```python
from build123d import *

# Parameters (mm, degrees)
SKETCH_1_R          = 9.1
EXTRUDE_1_DEPTH     = 64.7
FILLET_1_R          = 0.5
FILLET_2_R          = 0.5
SKETCH_2_R          = 6.5
CUT_EXTRUDE_1_DEPTH = 0.35
SKETCH_3_R          = 6.5
CUT_EXTRUDE_2_DEPTH = 0.35
SKETCH_4_R          = 4.25
EXTRUDE_2_DEPTH     = 0.8
FILLET_3_R          = 0.5
SKETCH_5_R          = 6.5
SKETCH_5_R_2        = 4.25
EXTRUDE_3_DEPTH     = 0.2


with BuildPart() as part:
    # 草图1 → 凸台-拉伸1 (new body)
    with BuildSketch(Plane.XY):
        with Locations((-28.874360447, 15.271996124)):
            Circle(SKETCH_1_R)
    extrude(amount=EXTRUDE_1_DEPTH)

    # 圆角1
    fillet_1_edges = [part.edges().sort_by_distance(p)[0] for p in [
        (-37.974360447, 15.271996124, 0),
    ]]
    fillet(fillet_1_edges, radius=FILLET_1_R)

    # 圆角2
    fillet_2_edges = [part.edges().sort_by_distance(p)[0] for p in [
        (-37.974360447, 15.271996124, 64.7),
    ]]
    fillet(fillet_2_edges, radius=FILLET_2_R)

    # 草图2 → 切除-拉伸1 (cut)
    with BuildSketch(Plane(origin=(0, 0, 0), x_dir=(-1, 0, 0), z_dir=(0, 0, -1))):
        with Locations((28.874360447, 15.271996124)):
            Circle(SKETCH_2_R)
    extrude(amount=-CUT_EXTRUDE_1_DEPTH, mode=Mode.SUBTRACT)

    # 草图3 → 切除-拉伸2 (cut)
    with BuildSketch(Plane.XY.offset(64.7)):
        with Locations((-28.874360447, 15.271996124)):
            Circle(SKETCH_3_R)
    extrude(amount=-CUT_EXTRUDE_2_DEPTH, mode=Mode.SUBTRACT)

    # 草图4 → 凸台-拉伸2 (add)
    with BuildSketch(Plane.XY.offset(64.35)):
        with Locations((-28.874360447, 15.271996124)):
            Circle(SKETCH_4_R)
    extrude(amount=EXTRUDE_2_DEPTH)

    # 圆角3
    fillet_3_edges = [part.edges().sort_by_distance(p)[0] for p in [
        (-33.124360447, 15.271996124, 65.15),
    ]]
    fillet(fillet_3_edges, radius=FILLET_3_R)

    # 草图5 → 凸台-拉伸3 (add)
    with BuildSketch(Plane.XY.offset(64.35)):
        with Locations((-28.874360447, 15.271996124)):
            Circle(SKETCH_5_R)
        with Locations((-28.874360447, 15.271996124)):
            Circle(SKETCH_5_R_2, mode=Mode.SUBTRACT)
    extrude(amount=EXTRUDE_3_DEPTH)


solid = part.part
```
Here's how the part is built. I have some questions about the finished solid (model axes, mm). A direction names the side the tool comes from. Round coordinates to 2 decimals unless told otherwise and drop trailing zeros. Order: outer loops, then holes, each group sorted by start corner. A loop starts at its lowest first (then second) coordinate and runs counter-clockwise, first axis right, second up. Notation, with made-up numbers: M 6,80.25 L 41,80.25 A29 ccw 41,111.25 Z; hole C -21,11 d7. An arc over 180 degrees is marked long. Answer in a Markdown table with one row per item.
Item 1: Imagine slicing it at A-A, the plane z = 49. Write out the boundary of the cut face in (x, y).
A:
| item | result |
|---|---|
| outline | C -28.87,15.27 d18.2 |
Item 2: Thinking about a two-plate mould opening in Y: for faces 4 (the face through (-37.966, 15.672, 31.904)), 5 (the face through (-29, 15, 0.35)), 6 (the face through (-29, 15, 65.15)), which applies, +Y half, -Y half, draft (parallel to the pull), parting line (faces both ways), or undercut?
A:
| item | result |
|---|---|
| face 4 | parting line |
| face 5 | undercut |
| face 6 | draft |
Item 3: For faces 1 (the face through (-28, 22, 0)), 2 (the face through (-22.38, 15.56, 0.17)), 3 (the face through (-28, 22, 64.7)), which set-ups out of +Z, -Z, +X, -X, +Y, -Y let a thin tool reach every point of the face, with its end or its side?
A:
| item | result |
|---|---|
| face 1 | -Z, +X, -X, +Y, -Y |
| face 2 | -Z |
| face 3 | +Z |
Item 4: If I drill on L1, parallel to Z at x = -26, y = 10; L2, parallel to Z at x = -31, y = 12.75; L3, parallel to Y at x = -22.5, z = 23.5, over which ranges is the centre line in solid material (lowest first)? Write a range as from..to.
A:
| item | result |
|---|---|
| L1 | z = 0.35..64.55 |
| L2 | z = 0.35..65.15 |
| L3 | y = 8.78..21.77 |
Item 5: I'm going to push flat-ended pins straight in: pin 1 (1 mm diameter, centred on y = 16, z = 33.5, fed in from -X); pin 2 (1 mm diameter, centred on y = 20.5, z = 49.5, fed in from +X); pin 3 (3 mm diameter, centred on y = 22.5, z = 53.5, fed in from -X); pin 4 (10.5 mm diameter, centred on x = -28.5, y = 13, fed in from -Z). Where does each tip first touch, or does it pass through?
A:
| item | result |
|---|---|
| pin 1 | stops at x = -37.97 |
| pin 2 | stops at x = -21.1 |
| pin 3 | stops at x = -35.95 |
| pin 4 | stops at z = 0 |
